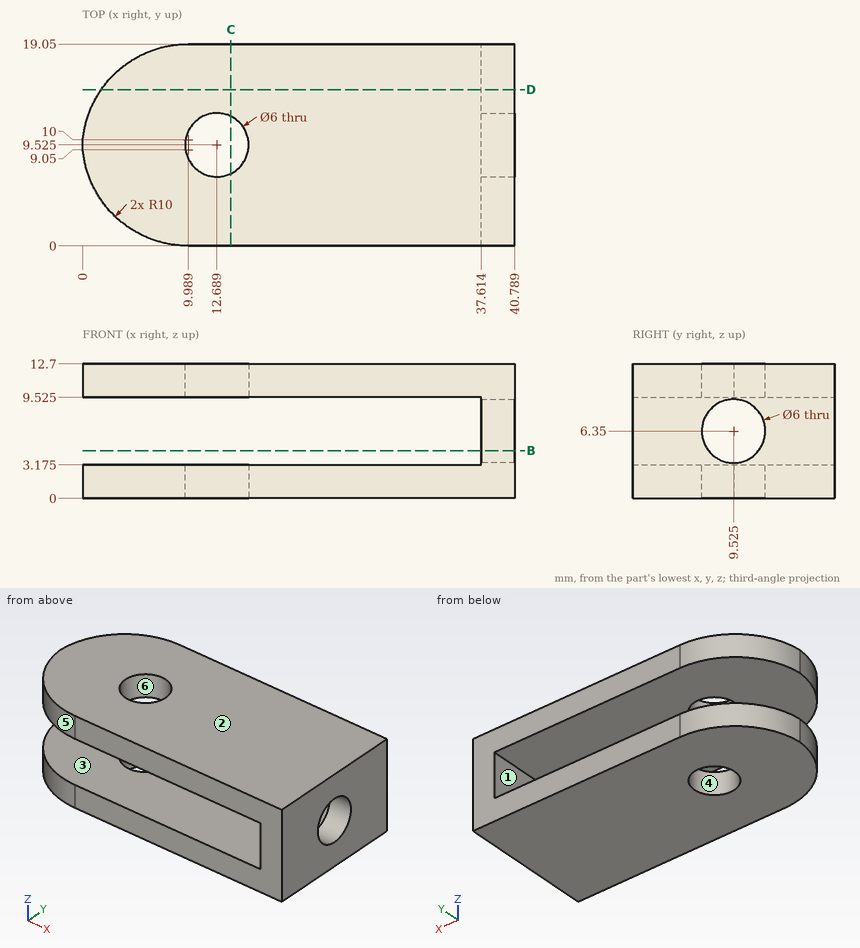
Can you work these out from the drawing? Everything is in mm from the part's minimum corner. A direction names the side the tool comes from. Give positions to 0.01 mm unless a question says otherwise; leave off trailing zeros. Write each loop counter-clockwise with the first axis right and the second up, starting at its lowest first coordinate (ties: lowest second). Pieces come first, ordered by that corner, then holes. Notation, with made-up numbers: M 7.5,-31 L 64.5,-31 A16 ccw 64.5,-20 Z; hole C -9,27.25 d3. An arc over 180 degrees is marked long. Answer in a Markdown table with one row per item. Add a question column.
Item 1: Imagine slicing it at B-B, the plane z = 4.5. Write out the boundary of the cut face in (x, y), plus the area to 3 significant figures.
Item 2: For pin 1 Ø1.5 at (x, z) = (31, 9) entering from -Y; pin 2 Ø1.9 at (y, z) = (10, 6) entering from -X; pin 3 Ø5 at (y, z) = (14, 1.5) entering from -X, each with a flat end and sliding along its axis, tell me the tip position at first contact or that it passes through.
Item 3: We'd pull the mould along X, two halves only. Please class the marked faces 3, 4, 5 and 6: released by +X, released by -X, zero draft, split by the parting line, or undercut.
Item 4: Please list where these lines run through material, in increasing order: L1, parallel to Z at x = 24.5, y = 8.5 (1 decimal); L2, parallel to X at y = 14, z = 5; L3, parallel to X at y = 12, z = 1 (1 decimal).
Item 5: On a 3-axis mill with a long thin cutter (end or side, diameter ignored), from which of +Z, -Z, +X, -X, +Y, -Y can I reach the whole of each face in a straight line? I mean the marked faces 1 and 2. Say none if no direction works.
Item 6: Imagine slicing it at C-C, the plane x = 14. State how many separate pieces and enclosed holes the cut face has, plus the area to 3 significant figures.
Item 7: Imagine slicing it at D-D, the plane y = 14.75. Write out the boundary of the cut face in (x, z) (1 decimal), plus the area to 3 significant figures.
Evaluation:
| question | item | result |
|---|---|---|
| 1 | outline | M 37.61,0 L 40.79,0 L 40.79,7.16 L 37.61,7.16 Z; M 37.61,11.89 L 40.79,11.89 L 40.79,19.05 L 37.61,19.05 Z |
| 1 | area | 45.5 mm² |
| 2 | pin 1 | stops at y = 0 |
| 2 | pin 2 | passes through |
| 2 | pin 3 | stops at x = 0.29 |
| 3 | face 3 | zero draft |
| 3 | face 4 | undercut |
| 3 | face 5 | released by -X |
| 3 | face 6 | undercut |
| 4 | L1 | z = 0 to 3.2, 9.5 to 12.7 |
| 4 | L2 | x = 37.61 to 40.79 |
| 4 | L3 | x = 0.4 to 11, 14.4 to 40.8 |
| 5 | face 1 | -X, +Y, -Y |
| 5 | face 2 | +Z, +X, -X, +Y, -Y |
| 6 | separate pieces | 4 |
| 6 | enclosed holes | 0 |
| 6 | area | 86.7 mm² |
| 7 | outline | M 1.8,0 L 40.8,0 L 40.8,12.7 L 1.8,12.7 L 1.8,9.5 L 37.6,9.5 L 37.6,3.2 L 1.8,3.2 Z |
| 7 | area | 268 mm² |
